Model file for the job. Use its own axes, mm. Coordinates: 2 decimals unless noted, no trailing zeros. Write each loop counter-clockwise with the first axis right and the second up, starting at its lowest first coordinate (ties: lowest second). Pieces come first, ordered by that corner, then holes. Notation, with made-up numbers: M -35.5,3.5 L -7.5,3.5 A8 ccw -7.5,12.5 Z; hole C -4,85.5 d6. An arc over 180 degrees is marked long. Answer in a Markdown table with one row per item. Add a question column.
```python
from build123d import *

# Parameters (mm, degrees)
SKETCH_1_W           = 220
SKETCH_1_H           = 35
EXTRUDE_1_DEPTH      = 4
CUT_EXTRUDE_1_DEPTH  = 10
CHAMFER_1_SIZE       = 5
EXTRUDE_2_DEPTH      = 4
EXTRUDE_3_DEPTH      = 4
EXTRUDE_4_DEPTH      = 4
EXTRUDE_7_DEPTH      = 4
FILLET_1_R           = 2
SKETCH_21_W          = 4
SKETCH_21_H          = 5
SKETCH_21_H_2        = 6.299038106
CUT_EXTRUDE_8_DEPTH  = 4
SKETCH_22_R          = 1.40240318
CUT_EXTRUDE_9_DEPTH  = 4
EXTRUDE_8_DEPTH      = 4
CUT_EXTRUDE_14_DEPTH = 10
CUT_EXTRUDE_15_DEPTH = 4
CHAMFER_2_SIZE       = 3
CHAMFER_2_SIZE2      = 2.344579619
SKETCH_29_W          = 6
SKETCH_29_H          = 5
SKETCH_29_W_2        = 10
SKETCH_29_W_3        = 4
SKETCH_29_H_2        = 12
CUT_EXTRUDE_16_DEPTH = 4
SKETCH_30_R          = 1.4
CUT_EXTRUDE_17_DEPTH = 4
EXTRUDE_9_DEPTH      = 4
SKETCH_35_R          = 44.644180149
CUT_EXTRUDE_19_DEPTH = 126.325939799
SKETCH_36_R          = 1.40240318
SKETCH_36_R_2        = 1.4
SKETCH_36_W          = 4
SKETCH_36_H          = 5
SKETCH_36_H_2        = 6.299038106
EXTRUDE_11_DEPTH     = 4


with BuildPart() as part:
    # 草图1 → 凸台-拉伸1 (new body)
    with BuildSketch(Plane.XY):
        Rectangle(SKETCH_1_W, SKETCH_1_H)
    extrude(amount=EXTRUDE_1_DEPTH)

    # 草图2 → 切除-拉伸1 (cut)
    with BuildSketch(Plane.XY.offset(4)):
        Polygon((0, 17.519994919), (-16.999988241, 17.5), (-16.999988241, 0), (17.000011759, 0), (17.000011759, 17.5), align=None)
    extrude(amount=-CUT_EXTRUDE_1_DEPTH, mode=Mode.SUBTRACT)

    # 倒角1
    chamfer_1_edges = [part.edges().sort_by_distance(p)[0] for p in [
        (17.000011759, 17.5, 2),
        (-16.999988241, 17.5, 2),
    ]]
    chamfer(chamfer_1_edges, length=CHAMFER_1_SIZE)

    # 草图3 → 凸台-拉伸2 (add)
    with BuildSketch(Plane(origin=(0, 0, 0), x_dir=(-1, 0, 0), z_dir=(0, 0, -1))):
        Polygon((-17.000011759, 0), (-17.000011759, 12.5), (-14.000011759, 0), align=None)
        Polygon((16.999988241, 12.5), (16.999988241, 0), (13.999988241, 0), align=None)
    extrude(amount=-EXTRUDE_2_DEPTH)

    # 草图4 → 凸台-拉伸3 (add)
    with BuildSketch(Plane(origin=(0, 0, 0), x_dir=(-1, 0, 0), z_dir=(0, 0, -1))):
        Polygon((-22.000011759, 17.5), (-29.071079571, 24.571067812), (-110, 17.5), align=None)
        Polygon((21.999988241, 17.5), (29.071056053, 24.571067812), (110, 17.5), align=None)
    extrude(amount=-EXTRUDE_3_DEPTH)

    # 草图7 → 凸台-拉伸4 (add)
    with BuildSketch(Plane(origin=(0, 0, 0), x_dir=(-1, 0, 0), z_dir=(0, 0, -1))):
        Polygon((-110, 17.5), (-115.977227757, 16.97774686), (-112.5, -17.5), (-110, -17.5), align=None)
    extrude_4 = extrude(amount=-EXTRUDE_4_DEPTH)

    # 草图19 → 凸台-拉伸7 (add)
    with BuildSketch(Plane(origin=(0, 0, 0), x_dir=(-1, 0, 0), z_dir=(0, 0, -1))):
        Polygon((-17.000011759, 12.5), (-29.071079571, 24.571067812), (-25.649595146, 25.392224074), (-14.280331934, 14.022960862), (-11.634821327, 3), (11.63479781, 3), (14.280308417, 14.022960862), (25.169324411, 24.911976857), (29.071056053, 24.571067812), (16.999988241, 12.5), (13.999988241, 0), (-14.000011759, 0), align=None)
    extrude(amount=-EXTRUDE_7_DEPTH)

    # 圆角1
    fillet_1_edges = [part.edges().sort_by_distance(p)[0] for p in [
        (-11.63479781, 3, 2),
        (11.634821327, 3, 2),
    ]]
    fillet(fillet_1_edges, radius=FILLET_1_R)

    # 草图21 → 切除-拉伸8 (cut)
    with BuildSketch(Plane(origin=(133.943153128, -40.880278438, 0), x_dir=(1, 0, 0), z_dir=(0, 0, -1))):
        with Locations((-67.143153128, -53.147127978)):
            Rectangle(SKETCH_21_W, SKETCH_21_H)
        with Locations((-74.143153128, -53.147127978)):
            Rectangle(SKETCH_21_W, SKETCH_21_H)
        with Locations((-67.143153128, -39.44868951)):
            Rectangle(SKETCH_21_W, SKETCH_21_H_2)
        with Locations((-74.143153128, -39.44868951)):
            Rectangle(SKETCH_21_W, SKETCH_21_H_2)
        with Locations((-109.943153128, -53.147127978)):
            Rectangle(SKETCH_21_W, SKETCH_21_H)
        with Locations((-109.943153128, -39.44868951)):
            Rectangle(SKETCH_21_W, SKETCH_21_H_2)
        with Locations((-157.943153128, -39.44868951)):
            Rectangle(SKETCH_21_W, SKETCH_21_H_2)
        with Locations((-157.943153128, -53.147127978)):
            Rectangle(SKETCH_21_W, SKETCH_21_H)
        with Locations((-200.743153128, -39.44868951)):
            Rectangle(SKETCH_21_W, SKETCH_21_H_2)
        with Locations((-193.743153128, -39.44868951)):
            Rectangle(SKETCH_21_W, SKETCH_21_H_2)
        with Locations((-193.743153128, -53.147127978)):
            Rectangle(SKETCH_21_W, SKETCH_21_H)
        with Locations((-200.743153128, -53.147127978)):
            Rectangle(SKETCH_21_W, SKETCH_21_H)
    extrude(amount=-CUT_EXTRUDE_8_DEPTH, mode=Mode.SUBTRACT)

    # 草图22 → 切除-拉伸9 (cut)
    with BuildSketch(Plane(origin=(133.943153128, -40.880278438, 0), x_dir=(1, 0, 0), z_dir=(0, 0, -1))):
        with Locations(Location((-109.943153128, -46.620265091, 0), (0, 0, 180))):
            Circle(SKETCH_22_R)
        with Locations(Location((-74.143153128, -46.620265091, 0), (0, 0, 180))):
            Circle(SKETCH_22_R)
        with Locations(Location((-67.143153128, -46.620265091, 0), (0, 0, 180))):
            Circle(SKETCH_22_R)
    cut_extrude_9 = extrude(amount=-CUT_EXTRUDE_9_DEPTH, mode=Mode.SUBTRACT)

    # 镜向10: 切除-拉伸9 across plane
    add(cut_extrude_9.mirror(Plane(origin=(0, 0, 0), x_dir=(0, 0, 1), z_dir=(1, 0, 0))), mode=Mode.SUBTRACT)

    # 镜向11: 凸台-拉伸4 across plane
    add(extrude_4.mirror(Plane(origin=(0, 0, 0), x_dir=(0, 0, 1), z_dir=(1, 0, 0))))

    # 草图23 → 凸台-拉伸8 (add)
    with BuildSketch(Plane(origin=(0, 0, 0), x_dir=(-1, 0, 0), z_dir=(0, 0, -1))):
        Polygon((115.977227757, 16.97774686), (112.5, -17.5), (123.677307019, -17.5), (127.041988649, 15.861818553), align=None)
    extrude(amount=-EXTRUDE_8_DEPTH)

    # 草图27 → 切除-拉伸14 (cut)
    with BuildSketch(Plane(origin=(0, 0, 0), x_dir=(-1, 0, 0), z_dir=(0, 0, -1))):
        Polygon((123.677307019, -17.5), (127.041988649, 15.861818553), (110.453235561, 19.244980627), (111.116335779, 17.402461494), align=None)
    extrude(amount=-CUT_EXTRUDE_14_DEPTH, mode=Mode.SUBTRACT)

    # 草图28 → 切除-拉伸15 (cut)
    with BuildSketch(Plane(origin=(133.943153128, -40.880278438, 0), x_dir=(1, 0, 0), z_dir=(0, 0, -1))):
        Polygon((-214.384814898, -36.029379852), (-223.826225744, -39.324795038), (-222.178518151, -44.04550046), (-212.737107305, -40.750085275), align=None)
        Polygon((-239.450613316, -34.009451966), (-237.802905723, -38.730157389), (-232.138059216, -36.752908277), (-233.785766808, -32.032202855), align=None)
        Polygon((-242.830523796, -45.567593925), (-246.785022019, -34.23790091), (-250.561586358, -35.556066985), (-246.607088135, -46.885759999), align=None)
    extrude(amount=-CUT_EXTRUDE_15_DEPTH, mode=Mode.SUBTRACT)

    # 倒角2
    chamfer_2_edges = [part.edges().sort_by_distance(p)[0] for p in [
        (-123.677307019, -17.5, 2),
    ]]
    chamfer_2_side = [part.faces().sort_by_distance(p)[0] for p in [
        (-117.396821399, -0.048769253, 2),
    ]]
    chamfer(chamfer_2_edges, length=CHAMFER_2_SIZE, length2=CHAMFER_2_SIZE2, reference=chamfer_2_side[0])

    # 草图29 → 切除-拉伸16 (cut)
    with BuildSketch(Plane(origin=(133.943153128, -40.880278438, 0), x_dir=(1, 0, 0), z_dir=(0, 0, -1))):
        with Locations((-37.943153128, -39.581582586)):
            Rectangle(SKETCH_29_W, SKETCH_29_H)
        with Locations((-52.943153128, -49.748900766)):
            Rectangle(SKETCH_29_W_2, SKETCH_29_H)
        with Locations((-25.943153128, -40.880278438)):
            Rectangle(SKETCH_29_W_3, SKETCH_29_H_2)
    extrude(amount=-CUT_EXTRUDE_16_DEPTH, mode=Mode.SUBTRACT)

    # 草图30 → 切除-拉伸17 (cut)
    with BuildSketch(Plane(origin=(133.943153128, -40.880278438, 0), x_dir=(1, 0, 0), z_dir=(0, 0, -1))):
        with Locations(Location((-39.943153128, -49.748900766, 0), (0, 0, 180))):
            Circle(SKETCH_30_R)
        with Locations(Location((-230.555500624, -44.321479898, 0), (0, 0, 180))):
            Circle(SKETCH_30_R)
    extrude(amount=-CUT_EXTRUDE_17_DEPTH, mode=Mode.SUBTRACT)

    # 草图31 → 凸台-拉伸9 (add)
    with BuildSketch(Plane(origin=(0, 0, 0), x_dir=(-1, 0, 0), z_dir=(0, 0, -1))):
        Polygon((111.116335769, 17.402461523), (114.104949654, 17.141335029), (122.661428914, -14.677236872), align=None)
    extrude(amount=-EXTRUDE_9_DEPTH)

    # 草图35 → 切除-拉伸19 (cut, through all)
    with BuildSketch(Plane(origin=(0, 0, 0), x_dir=(0, 0, -1), z_dir=(1, 0, 0))):
        Circle(SKETCH_35_R)
    extrude(amount=CUT_EXTRUDE_19_DEPTH, mode=Mode.SUBTRACT)

    # 草图36 → 凸台-拉伸11 (add)
    with BuildSketch(Plane(origin=(0, 0, 0), x_dir=(-1, 0, 0), z_dir=(0, 0, -1))):
        with BuildLine():
            Line((-121.3327274, -17.5), (121.3327274, -17.5))
            Line((121.3327274, -17.5), (122.661428914, -14.677236872))
            Line((122.661428914, -14.677236872), (114.104949654, 17.141335029))
            Line((114.104949654, 17.141335029), (110, 17.5))
            Line((110, 17.5), (25.169324411, 24.911976857))
            Line((25.169324411, 24.911976857), (14.280308417, 14.022960862))
            Line((14.280308417, 14.022960862), (12.002778792, 4.533254095))
            ThreePointArc((12.002778792, 4.533254095), (11.296250567, 3.429412242), (10.058004188, 3))
            Line((10.058004188, 3), (-10.058004188, 3))
            ThreePointArc((-10.058004188, 3), (-11.296250567, 3.429412242), (-12.002778792, 4.533254095))
            Line((-12.002778792, 4.533254095), (-14.280308417, 14.022960862))
            Line((-14.280308417, 14.022960862), (-25.169324411, 24.911976857))
            Line((-25.169324411, 24.911976857), (-110, 17.5))
            Line((-110, 17.5), (-114.104949654, 17.141335029))
            Line((-114.104949654, 17.141335029), (-122.661428914, -14.677236872))
            Line((-122.661428914, -14.677236872), (-121.3327274, -17.5))
        make_face()
        with Locations(Location((24, 5.739986652, 0), (0, 0, 180))):
            Circle(SKETCH_36_R, mode=Mode.SUBTRACT)
        with Locations(Location((59.8, 5.739986652, 0), (0, 0, 180))):
            Circle(SKETCH_36_R, mode=Mode.SUBTRACT)
        with Locations(Location((66.8, 5.739986652, 0), (0, 0, 180))):
            Circle(SKETCH_36_R, mode=Mode.SUBTRACT)
        with Locations((96.612347495, 3.44120146)):
            Circle(SKETCH_36_R_2, mode=Mode.SUBTRACT)
        with Locations(Location((-96.612347495, 3.44120146, 0), (0, 0, 180))):
            Circle(SKETCH_36_R_2, mode=Mode.SUBTRACT)
        with Locations(Location((-66.8, 5.739986652, 0), (0, 0, 180))):
            Circle(SKETCH_36_R, mode=Mode.SUBTRACT)
        with Locations(Location((-59.8, 5.739986652, 0), (0, 0, 180))):
            Circle(SKETCH_36_R, mode=Mode.SUBTRACT)
        with Locations(Location((-24, 5.739986652, 0), (0, 0, 180))):
            Circle(SKETCH_36_R, mode=Mode.SUBTRACT)
        with Locations((24, 12.26684954)):
            Rectangle(SKETCH_36_W, SKETCH_36_H, mode=Mode.SUBTRACT)
        with Locations((24, -1.431588928)):
            Rectangle(SKETCH_36_W, SKETCH_36_H_2, mode=Mode.SUBTRACT)
        Polygon((80.44166177, -4.850898586), (89.883072616, -1.5554834), (88.235365023, 3.165222022), (78.793954177, -0.130193163), align=None, mode=Mode.SUBTRACT)
        with Locations((59.8, -1.431588928)):
            Rectangle(SKETCH_36_W, SKETCH_36_H_2, mode=Mode.SUBTRACT)
        with Locations((59.8, 12.26684954)):
            Rectangle(SKETCH_36_W, SKETCH_36_H, mode=Mode.SUBTRACT)
        with Locations((66.8, 12.26684954)):
            Rectangle(SKETCH_36_W, SKETCH_36_H, mode=Mode.SUBTRACT)
        Polygon((112.841868891, -6.642377528), (116.618433229, -5.324211453), (112.663935006, 6.005481561), (108.887370668, 4.687315487), align=None, mode=Mode.SUBTRACT)
        Polygon((105.507460187, -6.870826472), (103.859752595, -2.150121049), (98.194906087, -4.127370161), (99.84261368, -8.848075584), align=None, mode=Mode.SUBTRACT)
        with Locations((66.8, -1.431588928)):
            Rectangle(SKETCH_36_W, SKETCH_36_H_2, mode=Mode.SUBTRACT)
        with Locations((-66.8, 12.26684954)):
            Rectangle(SKETCH_36_W, SKETCH_36_H, mode=Mode.SUBTRACT)
        with Locations((-66.8, -1.431588928)):
            Rectangle(SKETCH_36_W, SKETCH_36_H_2, mode=Mode.SUBTRACT)
        Polygon((-98.194906087, -4.127370161), (-99.84261368, -8.848075584), (-105.507460187, -6.870826472), (-103.859752595, -2.150121049), align=None, mode=Mode.SUBTRACT)
        Polygon((-108.887370668, 4.687315487), (-112.841868891, -6.642377528), (-116.618433229, -5.324211453), (-112.663935006, 6.005481561), align=None, mode=Mode.SUBTRACT)
        with Locations((-59.8, 12.26684954)):
            Rectangle(SKETCH_36_W, SKETCH_36_H, mode=Mode.SUBTRACT)
        with Locations((-59.8, -1.431588928)):
            Rectangle(SKETCH_36_W, SKETCH_36_H_2, mode=Mode.SUBTRACT)
        Polygon((-89.883072616, -1.5554834), (-88.235365023, 3.165222022), (-78.793954177, -0.130193163), (-80.44166177, -4.850898586), align=None, mode=Mode.SUBTRACT)
        with Locations((-24, -1.431588928)):
            Rectangle(SKETCH_36_W, SKETCH_36_H_2, mode=Mode.SUBTRACT)
        with Locations((-24, 12.26684954)):
            Rectangle(SKETCH_36_W, SKETCH_36_H, mode=Mode.SUBTRACT)
    extrude(amount=-EXTRUDE_11_DEPTH)


solid = part.part
```
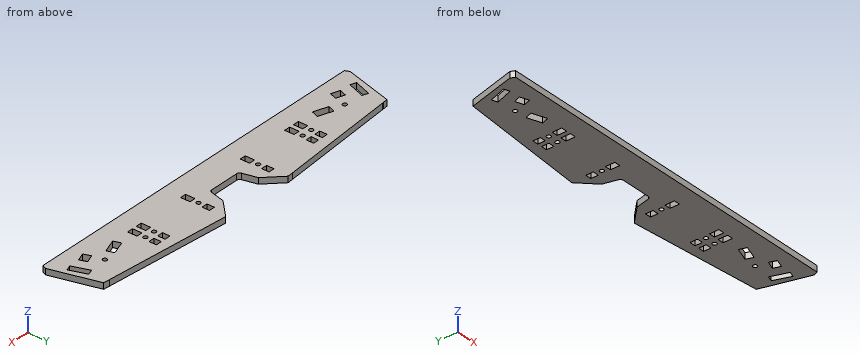
1) Drill centre lines: probe 1 along Y at (x, z) = (-66, 2.1); probe 2 along X at (y, z) = (3.5, 0.5); probe 3 along Y at (x, z) = (24, 3.2). Where is each one in solid material? Low to high.
2) Slice it at B-B (z = 2.25). Count the separate pieces of the cut face and the enclosed holes in it, then the cut area to 3 significant figures.
3) Slice it at C-C (x = 74). Give the cut face in (y, z), then the cut area to 3 significant figures.
4) Slice it at A-A (x = 39.5). Give the cut face in (y, z).
5) Flat gauge pins, fed straight in: pin 1 Ø1.2 at (x, z) = (24.5, 1) entering from +Y; pin 2 Ø1 at (x, z) = (-97, 3) entering from +Y; pin 3 Ø1.2 at (y, z) = (13, 1) entering from -X. Where does each tip first touch, or does it go through?
Ans:
| question | item | result |
|---|---|---|
| 1 | probe 1 | y = -17.5 to -4.58, 1.72 to 4.59, 6.89 to 9.77, 14.77 to 21.34 |
| 1 | probe 2 | x = -117.77 to -113.54, -109.3 to -98.01, -95.21 to -11.38, 11.38 to 95.21, 98.01 to 109.3, 113.54 to 117.77 |
| 1 | probe 3 | y = -17.5 to -4.58, 1.72 to 4.34, 7.14 to 9.77, 14.77 to 23.74 |
| 2 | separate pieces | 1 |
| 2 | enclosed holes | 26 |
| 2 | area | 8,010 mm2 |
| 3 | outline | M -17.5,0 L 20.65,0 L 20.65,4 L -17.5,4 Z |
| 3 | area | 153 mm2 |
| 4 | outline | M -17.5,0 L 23.66,0 L 23.66,4 L -17.5,4 Z |
| 5 | pin 1 | stops at y = 24.84 |
| 5 | pin 2 | stops at y = 18.68 |
| 5 | pin 3 | stops at x = -115.38 |
